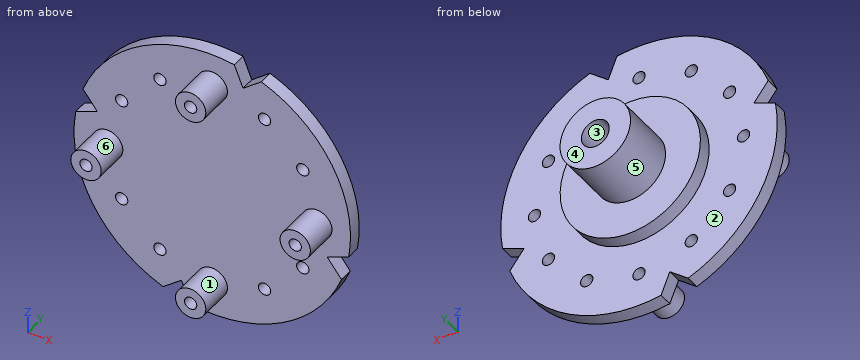
from build123d import *

# Parameters (mm, degrees)
SKETCH4_R           = 4.699
BOSS_EXTRUDE1_DEPTH = 10.668
SKETCH2_R           = 1.905
CUT_EXTRUDE1_DEPTH  = 65.262250988
CUT_EXTRUDE2_DEPTH  = 66.838691254


with BuildPart() as part:
    # Sketch1 → Revolve1 (revolve)
    with BuildSketch(Plane.XY, mode=Mode.PRIVATE) as revolve1_sk:
        Polygon((-42.799, 0), (0, 0), (0, 4.572), (-4.318, 4.572), (-4.318, 25.908), (-10.922, 25.908), (-10.922, 8.636), (-21.717, 8.636), (-21.717, 4.318), (-42.799, 4.318), align=None)
    revolve(revolve1_sk.sketch.rotate(Axis((0, 25.908, 0), (0, -1, 0)), 270), axis=Axis((0, 25.908, 0), (0, -1, 0)))

    # Sketch4 → Boss-Extrude1 (add)
    with BuildSketch(Plane.XZ):
        with Locations(Location((0, 32.385, 0), (0, 0, 90))):
            Circle(SKETCH4_R)
        with Locations(Location((32.385, 0, 0), (0, 0, 90))):
            Circle(SKETCH4_R)
        with Locations(Location((0, -32.385, 0), (0, 0, 90))):
            Circle(SKETCH4_R)
        with Locations(Location((-32.385, 0, 0), (0, 0, 90))):
            Circle(SKETCH4_R)
    extrude(amount=BOSS_EXTRUDE1_DEPTH)

    # Sketch2 → Cut-Extrude1 (cut, through all)
    with BuildSketch(Plane(origin=(0, 4.318, 0), x_dir=(1, 0, 0), z_dir=(0, 1, 0))):
        with Locations(Location((-32.385, 0, 0), (0, 0, 270))):
            Circle(SKETCH2_R)
        with Locations(Location((-28.046232702, 16.1925, 0), (0, 0, 270))):
            Circle(SKETCH2_R)
        with Locations(Location((-16.1925, 28.046232702, 0), (0, 0, 270))):
            Circle(SKETCH2_R)
        with Locations(Location((0, 32.385, 0), (0, 0, 270))):
            Circle(SKETCH2_R)
        with Locations(Location((16.1925, 28.046232702, 0), (0, 0, 270))):
            Circle(SKETCH2_R)
        with Locations(Location((28.046232702, 16.1925, 0), (0, 0, 270))):
            Circle(SKETCH2_R)
        with Locations(Location((32.385, 0, 0), (0, 0, 270))):
            Circle(SKETCH2_R)
        with Locations(Location((28.046232702, -16.1925, 0), (0, 0, 270))):
            Circle(SKETCH2_R)
        with Locations(Location((16.1925, -28.046232702, 0), (0, 0, 270))):
            Circle(SKETCH2_R)
        with Locations(Location((0, -32.385, 0), (0, 0, 270))):
            Circle(SKETCH2_R)
        with Locations(Location((-16.1925, -28.046232702, 0), (0, 0, 270))):
            Circle(SKETCH2_R)
        with Locations(Location((-28.046232702, -16.1925, 0), (0, 0, 270))):
            Circle(SKETCH2_R)
    extrude(amount=-CUT_EXTRUDE1_DEPTH, mode=Mode.SUBTRACT)

    # Sketch3 → Cut-Extrude2 (cut, through all)
    with BuildSketch(Plane.XZ):
        with BuildLine():
            Line((-35.575048182, 9.532305431), (-40.007033608, 15.204988091))
            ThreePointArc((-40.007033608, 15.204988091), (-41.340659439, 11.077196311), (-42.249601481, 6.835610853))
            Line((-42.249601481, 6.835610853), (-35.575048182, 9.532305431))
        make_face()
        with BuildLine():
            ThreePointArc((15.204988091, 40.007033608), (11.077196311, 41.340659439), (6.835610853, 42.249601481))
            Line((6.835610853, 42.249601481), (9.532305431, 35.575048182))
            Line((9.532305431, 35.575048182), (15.204988091, 40.007033608))
        make_face()
        with BuildLine():
            ThreePointArc((40.007033608, -15.204988091), (41.340659439, -11.077196311), (42.249601481, -6.835610853))
            Line((42.249601481, -6.835610853), (35.575048182, -9.532305431))
            Line((35.575048182, -9.532305431), (40.007033608, -15.204988091))
        make_face()
        with BuildLine():
            Line((-9.532305431, -35.575048182), (-15.204988091, -40.007033608))
            ThreePointArc((-15.204988091, -40.007033608), (-11.077196311, -41.340659439), (-6.835610853, -42.249601481))
            Line((-6.835610853, -42.249601481), (-9.532305431, -35.575048182))
        make_face()
    extrude(amount=-CUT_EXTRUDE2_DEPTH, mode=Mode.SUBTRACT)


solid = part.part
Verification items for the finished model (mm, model axes). Face numbers are marked on the shaded views. A direction names the side the tool comes from. Coordinates: 2 decimals unless noted, no trailing zeros. Order: outer loops, then holes, each group sorted by start corner. A loop starts at its lowest first (then second) coordinate and runs counter-clockwise, first axis right, second up.
1. Sectioned sample at A-A, the plane x = 0. Give the number of separate pieces and of enclosed holes in the cut face, and give its area (3 significant figures).
Results found:
separate pieces: 3
enclosed holes: 0
area: 837 mm2
2. Go/stop test with flat-tipped pins: pin 1 Ø1 at (x, z) = (-7.5, 11.5) entering from -Y; pin 2 Ø5 at (x, y) = (-3.5, 5) entering from +Z (3 decimals); pin 3 Ø5 at (x, z) = (0, -32.385) entering from +Y. Record where each tip stops, or that it passes through.
Results found:
pin 1: stops at y = 0
pin 2: stops at z = 42.785
pin 3: stops at y = 4.32
3. Release check for a two-part mould opening along X. For the marked faces 1, 2 and 3 record: +X half, -X half, draft (parallel to the pull), parting line (faces both ways), or undercut.
Results found:
face 1: parting line
face 2: draft
face 3: undercut
4. Sectioned sample at B-B, the plane y = -6. Record the cut outline in (x, z) (3 decimals), and give its area (3 significant figures).
Results found:
outline: circle Ø9.398 at (-32.385, 0); circle Ø9.398 at (0, -32.385); circle Ø9.398 at (0, 32.385); circle Ø9.398 at (32.385, 0); hole circle Ø3.81 at (-32.385, 0); hole circle Ø3.81 at (0, -32.385); hole circle Ø3.81 at (0, 32.385); hole circle Ø3.81 at (32.385, 0)
area: 232 mm2
5. Scan lines: line 1 (X direction, y = -2, z = 0); line 2 (X direction, y = 2, z = 27); line 3 (Y direction, x = -28.5, z = 30). Record each from-to range of solid material in increasing order.
Results found:
line 1: x = -37.08 to -34.29, -30.48 to -27.69, 27.69 to 30.48, 34.29 to 37.08
line 2: x = -33.21 to -17.78, -14.6 to 14.6, 17.78 to 33.21
line 3: y = 0 to 4.32
6. Sectioned sample at D-D, the plane x = -12. Record the cut outline in (y, z).
Results found:
outline: (0, -37.5) - (4.32, -37.5) - (4.32, -18.1) - (8.64, -18.1) - (8.64, 18.1) - (4.32, 18.1) - (4.32, 41.08) - (0, 41.08) - close
7. Set-up check for the marked faces 4, 5 and 6: record each of +Z, -Z, +X, -X, +Y, -Y from which the full face is reachable in a straight line by a thin tool's end or side.
Results found:
face 4: +Z, -Z, +X, -X, +Y
face 5: +Y
face 6: -Y
